Autodesk Inventor part; units mm, degrees
ref_plane "YZ Plane" through (0, 0, 0) normal (1, 0, 0) x (0, 1, 0)
ref_plane "XZ Plane" through (0, 0, 0) normal (0, 1, 0) x (-1, 0, 0)
ref_plane "XY Plane" through (0, 0, 0) normal (0, 0, 1) x (1, 0, 0)
sketch "Sketch1" plane through (0, 0, 0) normal (0, 1, 0) x (-1, 0, 0)
  line L0 (0, 0) -> (110, 0)
  line L1 (110, 0) -> (110, -85)
  line L2 (110, -85) -> (0, -85)
  line L3 (0, -85) -> (0, 0)
  dimension "d0" = 85
  dimension "d1" = 110
extrude "Extrusion1" add sketch "Sketch1" along normal blind 1.6
fillet "Fillet1" radius 5 4 edges at (0, 0.8, -85) (0, 0.8, 0) (-110, 0.8, 0) (-110, 0.8, -85)
sketch "Sketch2" plane through (0, 1.6, 0) normal (0, 1, 0) x (1, 0, 0)
  circle A0 centre (-4.3, 4) radius 1.95
  circle A1 centre (-4.3, 81) radius 1.95
  circle A2 centre (-105.7, 81) radius 1.95
  circle A3 centre (-105.7, 4) radius 1.95
  line L0 (-110, 80) -> (-110, 5)
  line L1 (-5, 85) -> (-105, 85)
  line L2 (-105, 0) -> (-5, 0)
  line L3 (0, 5) -> (0, 80)
  point P0 (0, 0)
  dimension "d5" = 3.9
  dimension "d6" = 3.9
  dimension "d7" = 3.9
  dimension "d8" = 3.9
  dimension "d9" = 4.3
  dimension "d10" = 4
  dimension "d11" = 4.3
  dimension "d12" = 4
  dimension "d13" = 4.3
  dimension "d14" = 4
  dimension "d15" = 4.3
  dimension "d16" = 4
extrude "Extrusion2" cut sketch "Sketch2" against normal through all
sketch "Sketch3" plane through (0, 1.6, 0) normal (0, 1, 0) x (1, 0, 0)
  circle A0 centre (-82.85, 19.05) radius 5.05
  circle A1 centre (-97.95, 19.05) radius 5.05
  line L0 (-105, 0) -> (-5, 0)
  line L1 (-110, 80) -> (-110, 5)
  point P0 (0, 0)
  dimension "d19" = 10.1
  dimension "d20" = 10.1
  dimension "d21" = 19.05
  dimension "d22" = 19.05
  dimension "d23" = 12.05
  dimension "d24" = 15.1
extrude "Extrusion3" add sketch "Sketch3" along normal blind 16
sketch "Sketch4" plane through (0, 1.6, 0) normal (0, 1, 0) x (1, 0, 0)
  line L0 (-14, 5) -> (-74, 5)
  line L1 (-74, 5) -> (-74, 32)
  line L2 (-74, 32) -> (-14, 32)
  line L3 (-14, 32) -> (-14, 5)
  line L4 (-105, 0) -> (-5, 0)
  line L5 (0, 5) -> (0, 80)
  point P0 (0, 0)
  dimension "d27" = 60
  dimension "d28" = 27
  dimension "d29" = 5
  dimension "d30" = 14
extrude "Extrusion4" add sketch "Sketch4" along normal blind 32
sketch "Sketch5" plane through (0, 1.6, 0) normal (0, 1, 0) x (1, 0, 0)
  line L0 (-81.5, 31) -> (-100.5, 31)
  line L1 (-100.5, 31) -> (-100.5, 74)
  line L2 (-100.5, 74) -> (-81.5, 74)
  line L3 (-81.5, 74) -> (-81.5, 31)
  line L4 (-110, 80) -> (-110, 5)
  line L5 (-5, 85) -> (-105, 85)
  point P0 (0, 0)
  dimension "d33" = 9.5
  dimension "d34" = 19
  dimension "d35" = 43
  dimension "d36" = 11
extrude "Extrusion5" add sketch "Sketch5" along normal blind 22
sketch "Sketch6" plane through (0, 1.6, 0) normal (0, 1, 0) x (1, 0, 0)
  line L0 (-49.5, 34) -> (-75.5, 34)
  line L1 (-75.5, 34) -> (-75.5, 46)
  line L2 (-75.5, 46) -> (-49.5, 46)
  line L3 (-49.5, 46) -> (-49.5, 34)
  line L4 (-74, 48) -> (-54, 48)
  line L5 (-54, 48) -> (-54, 76)
  line L6 (-54, 76) -> (-74, 76)
  line L7 (-74, 76) -> (-74, 48)
  line L8 (-13, 62.5) -> (-45, 62.5)
  line L9 (-45, 62.5) -> (-45, 76.5)
  line L10 (-45, 76.5) -> (-13, 76.5)
  line L11 (-13, 76.5) -> (-13, 62.5)
  line L12 (-12, 52) -> (-47, 52)
  line L13 (-47, 52) -> (-47, 62)
  line L14 (-47, 62) -> (-12, 62)
  line L15 (-12, 62) -> (-12, 52)
  line L16 (-12, 37) -> (-47, 37)
  line L17 (-47, 37) -> (-47, 47)
  line L18 (-47, 47) -> (-12, 47)
  line L19 (-12, 47) -> (-12, 37)
  line L20 (-5, 85) -> (-105, 85)
  line L21 (-81.5, 31) -> (-81.5, 74)
  line L22 (-14, 32) -> (-74, 32)
  line L23 (0, 5) -> (0, 80)
  point P0 (0, 0)
  dimension "d39" = 20
  dimension "d40" = 28
  dimension "d41" = 9
  dimension "d42" = 2
  dimension "d43" = 12
  dimension "d44" = 26
  dimension "d45" = 6
  dimension "d46" = 7.5
  dimension "d47" = 35
  dimension "d48" = 35
  dimension "d49" = 10
  dimension "d50" = 10
  dimension "d51" = 5
  dimension "d52" = 12
  dimension "d53" = 12
  dimension "d54" = 5
  dimension "d55" = 32
  dimension "d56" = 14
  dimension "d57" = 8.5
  dimension "d58" = 13
extrude "Extrusion6" add sketch "Sketch6" along normal blind 20 contours L7 L6 L5 L4
extrude "Extrusion7" add sketch "Sketch6" along normal blind 12 contours L0 L1 L2 L3
extrude "Extrusion8" add sketch "Sketch6" along normal blind 9.3 contours L12 L13 L14 L15 | L16 L17 L18 L19
extrude "Extrusion9" add sketch "Sketch6" along normal blind 14 contours L8 L9 L10 L11
equation "\"d6\" = d5"
equation "\"d7\" = d5"
equation "\"d8\" = d7"
equation "\"d11\" = d9"
equation "\"d12\" = d10"
equation "\"d13\" = d9"
equation "\"d14\" = d12"
equation "\"d15\" = d13"
equation "\"d16\" = d14"
equation "\"d19\" = d20"
equation "\"d22\" = d21"
equation "\"d48\" = d47"
equation "\"d50\" = d49"
equation "\"d53\" = d52"
properties part number "3waysplitter"
Could you check a few things on this model? Use its own coordinates, in mm. A direction names the side the tool comes from. Coordinates: 2 decimals unless noted, no trailing zeros. Order: outer loops, then holes, each group sorted by start corner. A loop starts at its lowest first (then second) coordinate and runs counter-clockwise, first axis right, second up.
Q1. Will these pins go through, and if not, where does the flat tip stop? pin 1 (10 mm diameter, centred on y = 7, z = -59, fed in from -X); pin 2 (1.5 mm diameter, centred on x = -12.5, y = 21.5, fed in from +Z); pin 3 (1 mm diameter, centred on x = -87, z = -45.5, fed in from +Y); pin 4 (3 mm diameter, centred on y = 22.5, z = -9, fed in from -X).
Q2. Which directions (+Z, -Z, +X, -X, +Y, -Y) give clear straight access to the entire face, cutting with the end or side of a thin tool? Please do faces 1 (the flat face through (-29, 9, -76.5)), 2 (the flat face through (-98, 17.6, -19)), 3 (the flat face through (-62, 8, -34)), 4 (the flat face through (-64, 21.6, -62)), 5 (the flat face through (-14, 17, -19)).
Q3. Thinking about a two-plate mould opening in X: for faces 6 (the flat face through (-100.5, 12, -52)), 7 (the cylindrical face through (-103.84, 0.81, -81.59)), 8 (the flat face through (-30, 10.9, -57)), which applies, released by +X, released by -X, zero draft, split by the parting line, or undercut?
Q4. Suppose I cut it at C-C on z = -19.05. Please give me the cut outline in (x, y).
Q5. Suppose I cut it at B-B on y = 8.5. Give the number of separate pieces and of enclosed holes in the cut face, and give its area (3 significant figures).
Q6. Suppose I cut it at A-A on y = 20. Please give me the cut outline in (x, z), and give its area (3 significant figures).
Q7. Please list where these lines run through material, in increasing order: L1, parallel to Z at x = -64, y = 12.5; L2, parallel to Z at x = -105.7, y = 0.8; L3, parallel to X at y = 0.4, z = -4.
Q8. Suppose I cut it at D-D on x = -26.5. Please give me the cut outline in (y, z).
Answer:
1. pin 1: stops at x = -100.5
1. pin 2: passes through
1. pin 3: stops at y = 23.6
1. pin 4: stops at x = -74
2. face 1: -Z, +X, -X, +Y
2. face 2: +Z, -X, +Y
2. face 3: +X, +Y
2. face 4: -Z, +X, +Y
2. face 5: +Z, +X, +Y
3. face 6: released by -X
3. face 7: undercut
3. face 8: zero draft
4. outline: (-110, 0) - (0, 0) - (0, 1.6) - (-14, 1.6) - (-14, 33.6) - (-74, 33.6) - (-74, 1.6) - (-77.8, 1.6) - (-77.8, 17.6) - (-87.9, 17.6) - (-87.9, 1.6) - (-92.9, 1.6) - (-92.9, 17.6) - (-103, 17.6) - (-103, 1.6) - (-110, 1.6) - close
5. separate pieces: 9
5. enclosed holes: 0
5. area: 4,620 mm2
6. outline: (-100.5, -74) - (-81.5, -74) - (-81.5, -31) - (-100.5, -31) - close; (-74, -76) - (-54, -76) - (-54, -48) - (-74, -48) - close; (-74, -32) - (-14, -32) - (-14, -5) - (-74, -5) - close
6. area: 3,000 mm2
7. L1: z = -76 to -48, -46 to -34, -32 to -5
7. L2: z = -84.95 to -82.95, -79.05 to -5.95, -2.05 to -0.05
7. L3: x = -109.9 to -107.65, -103.75 to -6.25, -2.35 to -0.1
8. outline: (0, -85) - (1.6, -85) - (1.6, -76.5) - (15.6, -76.5) - (15.6, -62.5) - (1.6, -62.5) - (1.6, -62) - (10.9, -62) - (10.9, -52) - (1.6, -52) - (1.6, -47) - (10.9, -47) - (10.9, -37) - (1.6, -37) - (1.6, -32) - (33.6, -32) - (33.6, -5) - (1.6, -5) - (1.6, 0) - (0, 0) - close
